For this review, take the finished solid that the model builds, in its own axes (mm). Face numbers are marked on the shaded views. A direction names the side the tool comes from. Give positions to 0.01 mm unless a question says otherwise; leave off trailing zeros. Write each loop counter-clockwise with the first axis right and the second up, starting at its lowest first coordinate (ties: lowest second). Pieces come first, ordered by that corner, then holes.
1) Wall thickness on line 1 along X through (y, z) = (-4, -0.05); line 2 along Y through (x, z) = (-0.1, -0.5); line 3 along Y through (x, z) = (0.45, -0.8): over which ranges is each line inside the solid? List them lowest first.
2) We need section A-A on z = 0. Give the boundary of the cut face in (x, y), and give its area (3 significant figures).
3) Machinability: for the marked faces 1 and 2, which of the approach directions +Z, -Z, +X, -X, +Y, -Y give a long, thin tool a straight path to every point of the face, cutting with its end or side? Answer none if there is none.
4) For P1, Ø1, axis at x = -0.5, y = -3, coming from the +Z side, flat-tipped, find the tip position at first contact; note if it passes through.
5) We need section B-B on y = -8. Give the boundary of the cut face in (x, z).
from build123d import *

# Parameters (mm, degrees)
F0_R          = 0.75
F1_DEPTH      = 10
F0_R_2        = 1
F2_DEPTH      = 0.25
F3_R          = 0.1
F5_DEPTH      = 25
F5_DEPTH_BACK = 25


with BuildPart() as f1:
    # F0 (on Front) → F1 (new body)
    with BuildSketch(Plane.XZ):
        Circle(F0_R)
    extrude(amount=F1_DEPTH)

    # F0 (on Front) → F2 (join)
    with BuildSketch(Plane.XZ):
        Circle(F0_R_2)
        Circle(F0_R, mode=Mode.SUBTRACT)
    extrude(amount=F2_DEPTH)

    # F3
    f3_edges = [f1.edges().sort_by_distance(p)[0] for p in [
        (-1, 0, 0),
    ]]
    fillet(f3_edges, radius=F3_R)

    # F4 (on Top) → F5 (cut, two sides)
    with BuildSketch(Plane.XY) as f5_sk:
        Polygon((-0.999971, -8.26199), (-0.999971, -10.461405), (0.999971, -10.461405), (0.999971, -8.26199), (0.799971, -8.26199), (0, -9.762005), (-0.799971, -8.26199), align=None)
    extrude(amount=F5_DEPTH, mode=Mode.SUBTRACT)
    extrude(f5_sk.sketch, amount=-F5_DEPTH_BACK, mode=Mode.SUBTRACT)


solid = f1.part
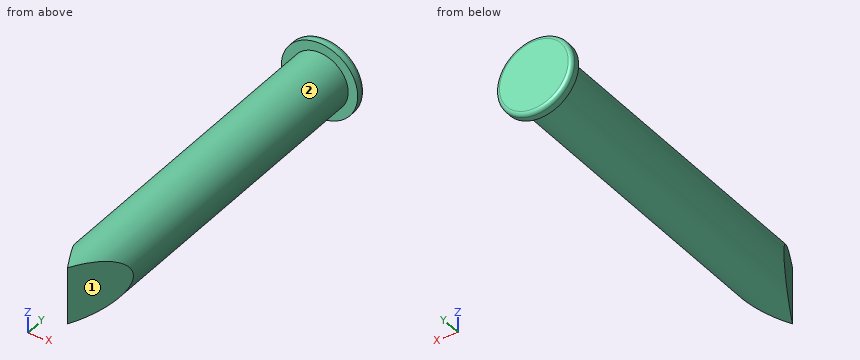
Results list:
1. line 1: x = -0.75 to 0.75
1. line 2: y = -9.57 to 0
1. line 3: y = -0.25 to 0
2. outline: (-1, -0.25) - (-0.75, -0.25) - (-0.75, -8.36) - (0, -9.76) - (0.75, -8.36) - (0.75, -0.25) - (1, -0.25) - (1, -0.1) arc R0.1 ccw to (0.9, 0) - (-0.9, 0) arc R0.1 ccw to (-1, -0.1) - close
2. area: 13.7 mm2
3. face 1: +Z, -Z, +X, -Y
3. face 2: -Y
4. P1: stops at z = 0.75
5. outline: circle Ø1.5 at (0, 0)
